Verification items for the finished model (mm, model axes). Face numbers are marked on the shaded views. A direction names the side the tool comes from. Give positions to 0.01 mm unless a question says otherwise; leave off trailing zeros. Order: outer loops, then holes, each group sorted by start corner. A loop starts at its lowest first (then second) coordinate and runs counter-clockwise, first axis right, second up. Notation, with made-up numbers: M 41,71.25 L 59,71.25 A19 ccw 59,92.25 Z; hole C 63,38.25 d4. An arc over 180 degrees is marked long. Answer as a JSON object with one key per item and string values.
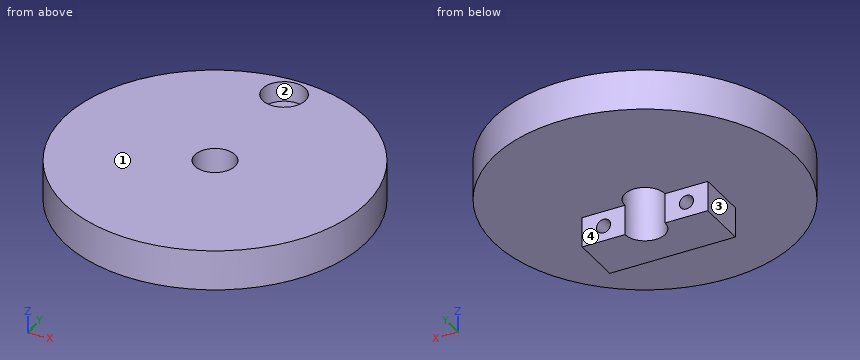
Autodesk Inventor part; units mm, degrees
ref_plane "YZ Plane" through (0, 0, 0) normal (1, 0, 0) x (0, 1, 0)
ref_plane "XZ Plane" through (0, 0, 0) normal (0, 1, 0) x (-1, 0, 0)
ref_plane "XY Plane" through (0, 0, 0) normal (0, 0, 1) x (1, 0, 0)
sketch "Sketch1" plane through (0, 0, 0) normal (0, 0, 1) x (1, 0, 0)
  circle A0 centre (0, 0) radius 30
  circle A1 centre (0, 0) radius 4
  dimension "d0" = 60
  dimension "d1" = 8
extrude "Extrusion1" add sketch "Sketch1" along normal blind 8
sketch "Sketch2" plane through (0, 0, 8) normal (0, 0, 1) x (1, 0, 0)
  circle A0 centre (0, 0) radius 30
  line L0 (0, 0) -> (0, 25) construction
  circle A1 centre (0, 25) radius 4.25
  dimension "d4" = 8.5
  dimension "d5" = 25
extrude "Extrusion2" cut sketch "Sketch2" against normal blind 4 contours A1
sketch "Sketch3" plane through (0, 0, 0) normal (0, 0, -1) x (-1, 0, 0)
  circle A0 centre (0, 0) radius 4
  line L0 (-4, 0) -> (-12.5, 0)
  line L1 (-12.5, 0) -> (-12.5, -10)
  line L2 (-12.5, -10) -> (12.5, -10)
  line L3 (12.5, -10) -> (12.5, 0)
  line L4 (12.5, 0) -> (4, 0)
  dimension "d8" = 10
  dimension "d9" = 25
extrude "Extrusion3" add sketch "Sketch3" along normal blind 6 contours L4 L3 L2 L1 L0 A0
sketch "Sketch4" plane through (4, 0, 0) normal (0, 1, 0) x (1, 0, 0)
  line L0 (8.5, 0) -> (0, 0)
  line L1 (0, 6) -> (8.5, 6)
  line L2 (-8, 0) -> (-16.5, 0)
  line L3 (-8, 0) -> (-8, 6)
  line L4 (-16.5, 6) -> (-8, 6)
  line L5 (-16.5, 0) -> (-16.5, 6)
  line L6 (-12.25, 6) -> (-12.25, 0) construction
  line L7 (4.25, 6) -> (4.25, 0) construction
  circle A0 centre (-12.25, 3) radius 1.4
  circle A1 centre (4.25, 3) radius 1.4
  point P0 (-4, 0)
  dimension "d12" = 2.8
extrude "Extrusion4" cut sketch "Sketch4" against normal through all contours A0 | A1
properties part number "sensor wheel"
Q1. Section check A-A on z = -3. Record the cut outline in (x, y), then the cut area to 3 significant figures.
Resolved:
{"outline": "M -12.5,-10 L -9.65,-10 L -9.65,0 L -12.5,0 Z; M -6.85,-10 L 6.85,-10 L 6.85,0 L 4,0 A4 cw -4,0 L -6.85,0 Z; M 9.65,-10 L 12.5,-10 L 12.5,0 L 9.65,0 Z", "area": "169 mm²"}
Q2. Material ranges on L1, parallel to X at y = -4.25, z = -3; L2, parallel to Y at x = 0, z = 3; L3, parallel to Z at x = 8.5, y = -20.5, recorded low to high.
Resolved:
{"L1": "x = -12.5 to -9.65, -6.85 to 6.85, 9.65 to 12.5", "L2": "y = -30 to -4, 4 to 30", "L3": "z = 0 to 8"}
Q3. Section check B-B on x = 0. Record the cut outline in (y, z), then the cut area to 3 significant figures.
Resolved:
{"outline": "M -30,0 L -10,0 L -10,-6 L -4,-6 L -4,8 L -30,8 Z; M 4,0 L 30,0 L 30,8 L 29.25,8 L 29.25,4 L 20.75,4 L 20.75,8 L 4,8 Z", "area": "418 mm²"}
Q4. Tool access check on the marked faces 1, 2, 3 and 4. Record the directions out of +Z, -Z, +X, -X, +Y, -Y that give a thin tool (end or side, any length) a straight path to the whole face; none if there is none.
Resolved:
{"face 1": "+Z, +X, -X, +Y, -Y", "face 2": "+Z", "face 3": "-Z, -X, +Y, -Y", "face 4": "-Z, +X, -X, +Y"}
Q5. Section check C-C on y = 21.5. Record the cut outline in (x, z), then the cut area to 3 significant figures.
Resolved:
{"outline": "M -20.92,0 L 20.92,0 L 20.92,8 L 2.41,8 L 2.41,4 L -2.41,4 L -2.41,8 L -20.92,8 Z", "area": "315 mm²"}
Q6. Gauge pin test, flat ends, axial feed: pin 1 Ø3 at (x, z) = (5.5, -4) entering from +Y; pin 2 Ø6.5 at (x, z) = (2, -4) entering from -Y; pin 3 Ø3 at (x, z) = (16, 2.5) entering from -Y. Record the tip position at first contact, or that the pin passes through.
Resolved:
{"pin 1": "stops at y = 0", "pin 2": "stops at y = -10", "pin 3": "stops at y = -26.26"}
Q7. Section check D-D on x = -11. Record the cut outline in (y, z).
Resolved:
{"outline": "M -27.91,0 L -10,0 L -10,-6 L 0,-6 L 0,0 L 27.91,0 L 27.91,8 L -27.91,8 Z"}
